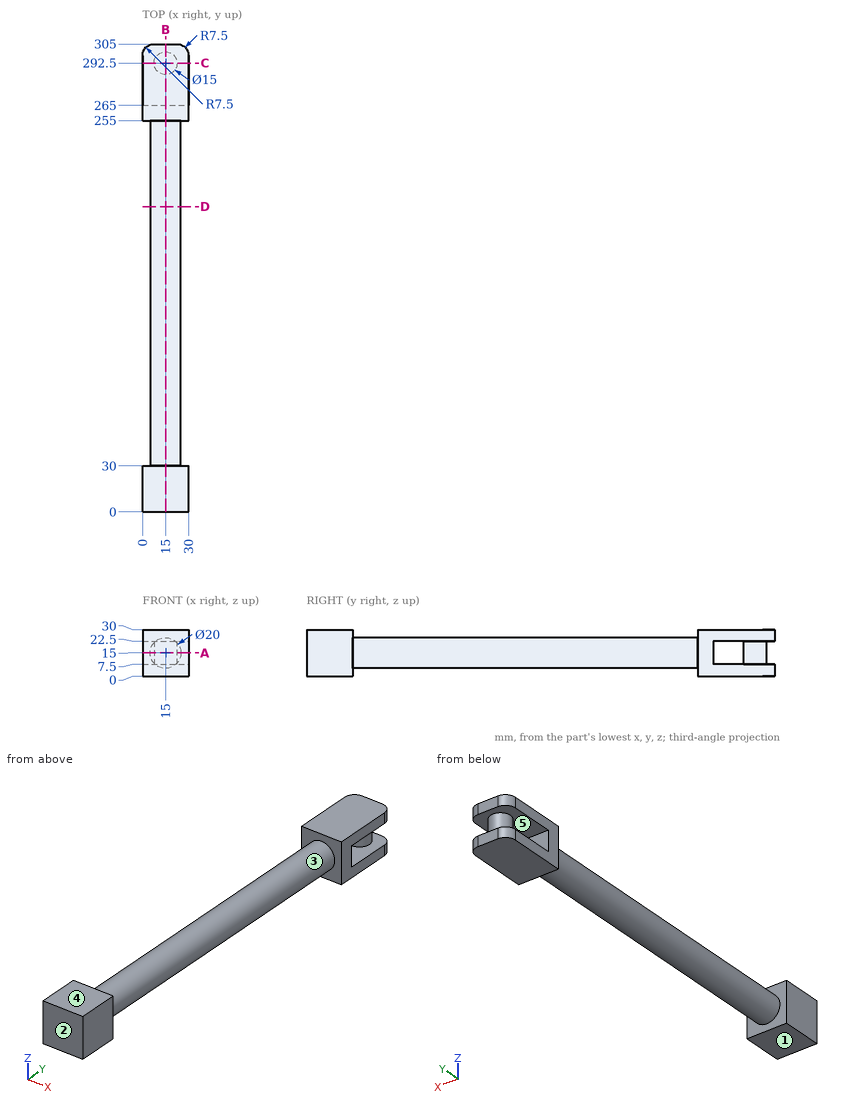
Part print with two shaded views. Sizes in mm from the minimum x, y, z corner. A direction names the side the tool comes from. Round coordinates to 2 decimals unless told otherwise and drop trailing zeros. Loops run counter-clockwise (first coordinate to the right, second up) from the corner with the lowest first, then second, coordinate; pieces in that order, holes last.
Item 1: Saw through at C-C (y = 292.5). List the corners of the cut face in (x, z), then the cut area to 3 significant figures.
Item 2: Saw through at A-A (z = 15). List the corners of the cut face in (x, y), then the cut area to 3 significant figures.
Item 3: Drill centre lines: line 1 along Y through (x, z) = (7, 8.25); line 2 along Y through (x, z) = (19, 2.5); line 3 along X through (y, z) = (199, 15.75). Where is each one in solid material? Low to high.
Item 4: Saw through at B-B (x = 15). List the corners of the cut face in (y, z).
Item 5: Saw through at D-D (y = 199). List the corners of the cut face in (x, z).
Item 6: Two-plate mould, pull along Y, no slides. Class the marked faces 1, 2 and 3: released by +Y, released by -Y, zero draft, split by the parting line, or undercut.
Item 7: Which spindle directions (+Z, -Z, +X, -X, +Y, -Y) get a long thin tool onto all of the face, cutting with end or side? Do the marked faces 4 and 5. Say none if no direction does.
Item 8: Pin check, flat tips, straight feed: P1, Ø2, axis at x = 18.5, y = 215, coming from the +Z side; P2, Ø5, axis at y = 72, z = 26.5, coming from the -X side; P3, Ø7.5, axis at x = 8.5, z = 13.5, coming from the +Y side. Stop position of each tip, or through.
Worked answers:
1. outline: (0, 0) - (30, 0) - (30, 7.5) - (22.5, 7.5) - (22.5, 22.5) - (30, 22.5) - (30, 30) - (0, 30) - (0, 22.5) - (7.5, 22.5) - (7.5, 7.5) - (0, 7.5) - close
1. area: 675 mm2
2. outline: (0, 0) - (30, 0) - (30, 30) - (25, 30) - (25, 255) - (30, 255) - (30, 265) - (0, 265) - (0, 255) - (5, 255) - (5, 30) - (0, 30) - close; circle Ø15 at (15, 292.5)
2. area: 5,880 mm2
3. line 1: y = 0 to 30, 255 to 265
3. line 2: y = 0 to 30, 255 to 305
3. line 3: x = 5.03 to 24.97
4. outline: (0, 0) - (30, 0) - (30, 5) - (255, 5) - (255, 0) - (305, 0) - (305, 7.5) - (300, 7.5) - (300, 22.5) - (305, 22.5) - (305, 30) - (255, 30) - (255, 25) - (30, 25) - (30, 30) - (0, 30) - close; hole (265, 7.5) - (285, 7.5) - (285, 22.5) - (265, 22.5) - close
5. outline: circle Ø20 at (15, 15)
6. face 1: zero draft
6. face 2: released by -Y
6. face 3: undercut
7. face 4: +Z, +X, -X, +Y, -Y
7. face 5: none
8. P1: stops at z = 24.68
8. P2: stops at x = 10.64
8. P3: stops at y = 299.48
